Design review of the part built by this model. Coordinates are the model's own, in mm. Coordinates: 2 decimals unless noted, no trailing zeros. Write each loop counter-clockwise with the first axis right and the second up, starting at its lowest first coordinate (ties: lowest second). Pieces come first, ordered by that corner, then holes. Notation, with made-up numbers: M 79.5,26.25 L 118.5,26.25 A18 ccw 118.5,44.25 Z; hole C 79,84 d2. An arc over 180 degrees is marked long. Write item = value, one per line.
```python
from build123d import *
from build123d.topology import SkipClean


with BuildPart() as part:
    # Sketch1 → Revolve1 (revolve)
    with SkipClean():  # the faces are left unmerged after this step: merging them gives an invalid solid
        with BuildSketch(Plane.XY, mode=Mode.PRIVATE) as revolve1_sk:
            with BuildLine():
                ThreePointArc((3.175, 0), (3.066814498, 0.821750468), (2.749630657, 1.5875))
                ThreePointArc((2.749630657, 1.5875), (-0.821750468, 3.066814498), (-3.175, 0))
                Line((-3.175, 0), (-1.5875, 0))
                ThreePointArc((-1.5875, 0), (0, 1.5875), (1.5875, 0))
                Line((1.5875, 0), (3.175, 0))
            make_face()
            with BuildLine():
                ThreePointArc((-3.175, 0), (0, -3.175), (3.175, 0))
                Line((3.175, 0), (1.5875, 0))
                ThreePointArc((1.5875, 0), (0, -1.5875), (-1.5875, 0))
                Line((-1.5875, 0), (-3.175, 0))
            make_face()
            with BuildLine():
                ThreePointArc((-1.5875, 0), (0, -1.5875), (1.5875, 0))
                Line((1.5875, 0), (-1.5875, 0))
            make_face()
            with BuildLine():
                Line((-1.5875, 0), (1.5875, 0))
                ThreePointArc((1.5875, 0), (0, 1.5875), (-1.5875, 0))
            make_face()
            with BuildLine():
                Line((117.900369343, 1.5875), (2.749630657, 1.5875))
                ThreePointArc((2.749630657, 1.5875), (3.066814498, 0.821750468), (3.175, 0))
                Line((3.175, 0), (117.475, 0))
                ThreePointArc((117.475, 0), (117.583185502, 0.821750468), (117.900369343, 1.5875))
            make_face()
            with BuildLine():
                ThreePointArc((119.0625, 0), (120.65, -1.5875), (122.2375, 0))
                Line((122.2375, 0), (119.0625, 0))
            make_face()
            with BuildLine():
                Line((119.0625, 0), (122.2375, 0))
                ThreePointArc((122.2375, 0), (120.65, 1.5875), (119.0625, 0))
            make_face()
            with BuildLine():
                ThreePointArc((123.825, 0), (121.471750468, 3.066814498), (117.900369343, 1.5875))
                ThreePointArc((117.900369343, 1.5875), (117.583185502, 0.821750468), (117.475, 0))
                Line((117.475, 0), (119.0625, 0))
                ThreePointArc((119.0625, 0), (120.65, 1.5875), (122.2375, 0))
                Line((122.2375, 0), (123.825, 0))
            make_face()
            with BuildLine():
                ThreePointArc((117.475, 0), (120.65, -3.175), (123.825, 0))
                Line((123.825, 0), (122.2375, 0))
                ThreePointArc((122.2375, 0), (120.65, -1.5875), (119.0625, 0))
                Line((119.0625, 0), (117.475, 0))
            make_face()
        revolve(revolve1_sk.sketch.rotate(Axis((123.825, 0, 0), (-1, 0, 0)), 90), axis=Axis((123.825, 0, 0), (-1, 0, 0)))

    # Boss-Extrude1: read off the stored shape, not the designer's step
    # Boss-Extrude1: loft between two sections, ruled curve by curve
    with SkipClean():  # the faces are left unmerged after this step: merging them gives an invalid solid
        boss_extrude1_from = [
            Edge.make_three_point_arc((119.0625, 0, 5.55625), (120.65, 1.5875, 5.55625), (122.2375, 0, 5.55625)),
            Edge.make_three_point_arc((122.2375, 0, 5.55625), (120.65, -1.5875, 5.55625), (119.0625, 0, 5.55625)),
        ]
        boss_extrude1_to = [
            Edge.make_three_point_arc((119.0625, 0, 2.749630657), (120.65, 1.5875, 2.749630657), (122.2375, 0, 2.749630657)),
            Edge.make_three_point_arc((122.2375, 0, 2.749630657), (120.65, -1.5875, 2.749630657), (119.0625, 0, 2.749630657)),
        ]
        boss_extrude1 = Solid(Shell([*[Face.make_surface_from_curves(boss_extrude1_from[k], boss_extrude1_to[k]) for k in range(2)], Face(Wire(boss_extrude1_from)), Face(Wire(boss_extrude1_to))]))
        add(boss_extrude1)

    # Boss-Extrude1 2: loft between two sections, ruled curve by curve
    with SkipClean():  # the faces are left unmerged after this step: merging them gives an invalid solid
        boss_extrude1_2_from = [
            Edge.make_three_point_arc((-1.5875, 0, 5.55625), (0, 1.5875, 5.55625), (1.5875, 0, 5.55625)),
            Edge.make_three_point_arc((1.5875, 0, 5.55625), (0, -1.5875, 5.55625), (-1.5875, 0, 5.55625)),
        ]
        boss_extrude1_2_to = [
            Edge.make_three_point_arc((-1.5875, 0, 2.749630657), (0, 1.5875, 2.749630657), (1.5875, 0, 2.749630657)),
            Edge.make_three_point_arc((1.5875, 0, 2.749630657), (0, -1.5875, 2.749630657), (-1.5875, 0, 2.749630657)),
        ]
        boss_extrude1_2 = Solid(Shell([*[Face.make_surface_from_curves(boss_extrude1_2_from[k], boss_extrude1_2_to[k]) for k in range(2)], Face(Wire(boss_extrude1_2_from)), Face(Wire(boss_extrude1_2_to))]))
        add(boss_extrude1_2)

    # Boss-Extrude1 3: loft between two sections, ruled curve by curve
    with SkipClean():  # the faces are left unmerged after this step: merging them gives an invalid solid
        boss_extrude1_3_from = [
            Edge.make_three_point_arc((122.2375, 0, -2.749630657), (120.65, -1.5875, -2.749630657), (119.0625, 0, -2.749630657)),
            Edge.make_three_point_arc((119.0625, 0, -2.749630657), (120.65, 1.5875, -2.749630657), (122.2375, 0, -2.749630657)),
        ]
        boss_extrude1_3_to = [
            Edge.make_three_point_arc((122.2375, 0, -5.55625), (120.65, -1.5875, -5.55625), (119.0625, 0, -5.55625)),
            Edge.make_three_point_arc((119.0625, 0, -5.55625), (120.65, 1.5875, -5.55625), (122.2375, 0, -5.55625)),
        ]
        boss_extrude1_3 = Solid(Shell([*[Face.make_surface_from_curves(boss_extrude1_3_from[k], boss_extrude1_3_to[k]) for k in range(2)], Face(Wire(boss_extrude1_3_from)), Face(Wire(boss_extrude1_3_to))]))
        add(boss_extrude1_3)

    # Boss-Extrude1 4: loft between two sections, ruled curve by curve
    with SkipClean():  # the faces are left unmerged after this step: merging them gives an invalid solid
        boss_extrude1_4_from = [
            Edge.make_three_point_arc((1.5875, 0, -2.749630657), (0, -1.5875, -2.749630657), (-1.5875, 0, -2.749630657)),
            Edge.make_three_point_arc((-1.5875, 0, -2.749630657), (0, 1.5875, -2.749630657), (1.5875, 0, -2.749630657)),
        ]
        boss_extrude1_4_to = [
            Edge.make_three_point_arc((1.5875, 0, -5.55625), (0, -1.5875, -5.55625), (-1.5875, 0, -5.55625)),
            Edge.make_three_point_arc((-1.5875, 0, -5.55625), (0, 1.5875, -5.55625), (1.5875, 0, -5.55625)),
        ]
        boss_extrude1_4 = Solid(Shell([*[Face.make_surface_from_curves(boss_extrude1_4_from[k], boss_extrude1_4_to[k]) for k in range(2)], Face(Wire(boss_extrude1_4_from)), Face(Wire(boss_extrude1_4_to))]))
        add(boss_extrude1_4)


solid = part.part
```
Q1. For P1, Ø3, axis at x = 49, z = 2.5, coming from the -Y side; P2, Ø1.5, axis at y = 2, z = 1.5, coming from the -X side, all flat-tipped, find the tip position at first contact; note any pin that passes through.
Check result:
P1 = -1.23
P2 = -2.65
Q2. Consider section B-B, the plane x = 100. State the section outline as (y, z) points (1 decimal), and give its area (3 significant figures).
Check result:
outline = C 0,0 d3.2
area = 7.92 mm²
Q3. Wall thickness on line 1 (X direction, y = -0.75, z = -2); line 2 (Z direction, x = 86.5, y = -0.25); line 3 (Y direction, x = 105.5, z = 0): over which ranges is each line inside the solid? List them lowest first.
Check result:
line_1 = -2.35 to 2.35, 118.3 to 123
line_2 = -1.57 to 1.57
line_3 = -1.59 to 1.59
Q4. The part is to be moulded in two halves that separate along X. For faces 1 (the cylindrical face through (59.519, 0.966, 1.26)), 2 (the flat face through (0, 0, -5.556)), say which applies: +X half, -X half, draft (parallel to the pull), parting line (faces both ways), or undercut.
Check result:
face_1 = undercut
face_2 = draft
